```python
from build123d import *

# Parameters (mm, degrees)
SKETCH1_R           = 80
SKETCH1_R_2         = 6
BOSS_EXTRUDE1_DEPTH = 13
SKETCH2_R           = 65
CUT_EXTRUDE1_DEPTH  = 8
SKETCH3_R           = 13
SKETCH3_R_2         = 6
BOSS_EXTRUDE2_DEPTH = 18
CHAMFER1_SIZE       = 1
CUT_EXTRUDE2_DEPTH  = 116.451288429
CIRPATTERN1_COUNT   = 10


with BuildPart() as part:
    # Sketch1 → Boss-Extrude1 (new, symmetric)
    with BuildSketch(Plane.XY):
        with Locations(Location((0, 0, 0), (0, 0, 180))):
            Circle(SKETCH1_R)
        with Locations(Location((0, 0, 0), (0, 0, 180))):
            Circle(SKETCH1_R_2, mode=Mode.SUBTRACT)
    extrude(amount=BOSS_EXTRUDE1_DEPTH, both=True)

    # Sketch2 → Cut-Extrude1 (cut)
    with BuildSketch(Plane.XY.offset(13)):
        Circle(SKETCH2_R)
    cut_extrude1 = extrude(amount=-CUT_EXTRUDE1_DEPTH, mode=Mode.SUBTRACT)

    # Mirror1: Cut-Extrude1 across plane
    add(cut_extrude1.mirror(Plane.XY), mode=Mode.SUBTRACT)

    # Sketch3 → Boss-Extrude2 (add, symmetric)
    with BuildSketch(Plane.XY):
        with Locations(Location((0, 0, 0), (0, 0, 180))):
            Circle(SKETCH3_R)
        with Locations(Location((0, 0, 0), (0, 0, 180))):
            Circle(SKETCH3_R_2, mode=Mode.SUBTRACT)
    extrude(amount=BOSS_EXTRUDE2_DEPTH, both=True)

    # Chamfer1
    chamfer1_edges = [part.edges().sort_by_distance(p)[0] for p in [
        (-65, 0, 13),
        (-65, 0, -13),
        (80, 0, -13),
        (80, 0, 13),
    ]]
    chamfer(chamfer1_edges, length=CHAMFER1_SIZE)

    # Sketch7 → Cut-Extrude2 (cut, through all)
    with BuildSketch(Plane.XY.offset(5)):
        with BuildLine():
            Line((0, 54.772255751), (0, 19.397164741))
            ThreePointArc((0, 19.397164741), (-0.515032591, 18.057436487), (-1.794871795, 17.407711947))
            ThreePointArc((-1.794871795, 17.407711947), (-4.529333289, 16.90370196), (-7.149451403, 15.972956666))
            ThreePointArc((-7.149451403, 15.972956666), (-8.582686936, 15.895715021), (-9.698582371, 16.798437427))
            Line((-9.698582371, 16.798437427), (-27.386127875, 47.434164903))
            ThreePointArc((-27.386127875, 47.434164903), (-27.821744262, 51.446675992), (-25.152000934, 54.473634439))
            ThreePointArc((-25.152000934, 54.473634439), (-15.529142706, 57.955549577), (-5.454545455, 59.751551728))
            ThreePointArc((-5.454545455, 59.751551728), (-1.629000688, 58.46500048), (0, 54.772255751))
        make_face()
    cut_extrude2 = extrude(amount=-CUT_EXTRUDE2_DEPTH, mode=Mode.SUBTRACT)

    # CirPattern1: Cut-Extrude2 ×10 about axis
    cirpattern1_axis = Axis((0, 0, 0), (0, 0, 1))
    for i in range(1, CIRPATTERN1_COUNT):
        add(cut_extrude2.rotate(cirpattern1_axis, i * 360 / CIRPATTERN1_COUNT), mode=Mode.SUBTRACT)


solid = part.part
```
Work out the finished part from the listing and answer in its coordinate system (mm). Coordinates: 2 decimals unless noted, no trailing zeros.
Q1. Each of these flat-tipped pins is pushed along its axis until it touches: pin 1 Ø1.5 at (x, y) = (55.5, 11.5) entering from -Z; pin 2 Ø11 at (y, z) = (-33.5, 1.5) entering from +X; pin 3 Ø5 at (y, z) = (-57.5, -11.5) entering from -X. Where does it stop, or does it pass through?
Q2. Find the intervals of material crossed by line 1 (Y direction, x = 0, z = 10); line 2 (Y direction, x = 50, z = -0.5); line 3 (Z direction, x = 41.5, y = 61), in increasing order.
Q3. A cutting plane is placed at A-A, the plane y = 0. State how many separate pieces and enclosed holes the cut face has, then the cut area to 3 significant figures.
Q4. Determine the mould class of faces 1 (the face through (-35.51, 11.54, 0.07)), 2 (the face through (-14.698, -9.498, 0.07)) for opening direction Y: released by +Y, released by -Y, zero draft, split by the parting line, or undercut.
Findings below:
1. pin 1: stops at z = -5
1. pin 2: stops at x = 74.94
1. pin 3: stops at x = -58.09
2. line 1: y = -80 to -65, -13 to -6, 6 to 13, 65 to 80
2. line 2: y = -62.45 to -33.17, -22.26 to -16.25, 10.63 to 16.25, 33.17 to 62.45
2. line 3: z = -13 to 13
3. separate pieces: 4
3. enclosed holes: 0
3. area: 1,470 mm2
4. face 1: undercut
4. face 2: undercut
